```python
from build123d import *

# Parameters (mm, degrees)
SKETCH1_R           = 0.9
BOSS_EXTRUDE1_DEPTH = 2


with BuildPart() as part:
    # Sketch1 → Boss-Extrude1 (new body)
    with BuildSketch(Plane.XY):
        with BuildLine():
            Line((16.2, 5), (16.2, 2))
            ThreePointArc((16.2, 2), (15.614213562, 0.585786438), (14.2, 0))
            Line((14.2, 0), (2, 0))
            ThreePointArc((2, 0), (0.585786438, 0.585786438), (0, 2))
            Line((0, 2), (0, 5))
            Line((0, 5), (4, 5))
            Line((4, 5), (4, 7))
            Line((4, 7), (0, 7))
            Line((0, 7), (0, 16.525))
            Line((0, 16.525), (4, 16.525))
            Line((4, 16.525), (4, 18.525))
            Line((4, 18.525), (0, 18.525))
            Line((0, 18.525), (0, 21.525))
            ThreePointArc((0, 21.525), (0.585786438, 22.939213562), (2, 23.525))
            Line((2, 23.525), (14.2, 23.525))
            ThreePointArc((14.2, 23.525), (15.614213562, 22.939213562), (16.2, 21.525))
            Line((16.2, 21.525), (16.2, 18.525))
            Line((16.2, 18.525), (12.2, 18.525))
            Line((12.2, 18.525), (12.2, 16.525))
            Line((12.2, 16.525), (16.2, 16.525))
            Line((16.2, 16.525), (16.2, 7))
            Line((16.2, 7), (12.2, 7))
            Line((12.2, 7), (12.2, 5))
            Line((12.2, 5), (16.2, 5))
        make_face()
        with Locations((13.45, 2.5)):
            Circle(SKETCH1_R, mode=Mode.SUBTRACT)
        with Locations((2.75, 21.025)):
            Circle(SKETCH1_R, mode=Mode.SUBTRACT)
        with Locations((13.45, 21.025)):
            Circle(SKETCH1_R, mode=Mode.SUBTRACT)
        with Locations((2.75, 2.5)):
            Circle(SKETCH1_R, mode=Mode.SUBTRACT)
    extrude(amount=BOSS_EXTRUDE1_DEPTH)


solid = part.part
```
Could you check a few things on this model? Use its own coordinates, in mm. A direction names the side the tool comes from. Coordinates: 2 decimals unless noted, no trailing zeros. Write each loop counter-clockwise with the first axis right and the second up, starting at its lowest first coordinate (ties: lowest second). Pieces come first, ordered by that corner, then holes. Notation, with made-up numbers: (48, 11) -> (65, 11) arc R27 cw to (65, 34) -> close; hole circle Ø11 at (89, -23.5). An arc over 180 degrees is marked (long way). Write item = value, one per line. Start each with the question number.
(1) I want a section at A-A (x = 2.75). Please give me the cut outline in (y, z) (3 decimals).
(2) Will this pin go through, and if not, where does the flat tip stop? pin 1 (0.6 mm diameter, centred on x = 15, z = 1, fed in from -Y).
(3) I need wall thicknesses on line 1 (Y direction, x = 13.45, z = 1.05) (3 decimals); line 2 (X direction, y = 20.5, z = 0.8); line 3 (Y direction, x = 3.5, z = 1.8) (1 decimal). Which ranges of each line are inside material? Lowest first, please. Write a range as [from, to].
(4) We'd pull the mould along X, two halves only. Please class faces 4 (the face through (2, 5, 1)), 5 (the face through (4, 18, 1)), 6 (the face through (12.2, 6, 1)), 7 (the face through (14.3, 2.2, 1)): released by +X, released by -X, zero draft, split by the parting line, or undercut.
(5) I want a section at D-D (x = 15). Please give me the cut outline in (y, z) (3 decimals), plus the area to 3 significant figures.
(6) Which directions (+Z, -Z, +X, -X, +Y, -Y) give clear straight access to the entire face, cutting with the end or side of a thin tool? Please do faces 1 (the face through (0.57, 22.924, 0.986)), 2 (the face through (2, 18.525, 1)), 3 (the face through (14, 16.525, 1)).
(7) I want a section at B-B (y = 2.5). Please give me the cut outline in (x, z).
(8) I want a section at C-C (z = 1.1). Please give me the cut outline in (x, y) (3 decimals).
Result set:
q1.outline = (0, 0) -> (1.6, 0) -> (1.6, 2) -> (0, 2) -> close; (3.4, 0) -> (5, 0) -> (5, 2) -> (3.4, 2) -> close; (7, 0) -> (16.525, 0) -> (16.525, 2) -> (7, 2) -> close; (18.525, 0) -> (20.125, 0) -> (20.125, 2) -> (18.525, 2) -> close; (21.925, 0) -> (23.525, 0) -> (23.525, 2) -> (21.925, 2) -> close
q2.pin_1 = 0.06
q3.line_1 = [0, 1.6], [3.4, 5], [7, 16.525], [18.525, 20.125], [21.925, 23.525]
q3.line_2 = [0, 2.02], [3.48, 12.72], [14.18, 16.2]
q3.line_3 = [0, 2], [3, 5], [7, 16.5], [18.5, 20.5], [21.5, 23.5]
q4.face_4 = zero draft
q4.face_5 = released by -X
q4.face_6 = released by +X
q4.face_7 = undercut
q5.outline = (0.167, 0) -> (5, 0) -> (5, 2) -> (0.167, 2) -> close; (7, 0) -> (16.525, 0) -> (16.525, 2) -> (7, 2) -> close; (18.525, 0) -> (23.358, 0) -> (23.358, 2) -> (18.525, 2) -> close
q5.area = 38.4 mm2
q6.face_1 = +Z, -Z, -X, +Y
q6.face_2 = +Z, -Z, -X
q6.face_3 = +Z, -Z, +X
q7.outline = (0, 0) -> (1.85, 0) -> (1.85, 2) -> (0, 2) -> close; (3.65, 0) -> (12.55, 0) -> (12.55, 2) -> (3.65, 2) -> close; (14.35, 0) -> (16.2, 0) -> (16.2, 2) -> (14.35, 2) -> close
q8.outline = (0, 2) arc R2 ccw to (2, 0) -> (14.2, 0) arc R2 ccw to (16.2, 2) -> (16.2, 5) -> (12.2, 5) -> (12.2, 7) -> (16.2, 7) -> (16.2, 16.525) -> (12.2, 16.525) -> (12.2, 18.525) -> (16.2, 18.525) -> (16.2, 21.525) arc R2 ccw to (14.2, 23.525) -> (2, 23.525) arc R2 ccw to (0, 21.525) -> (0, 18.525) -> (4, 18.525) -> (4, 16.525) -> (0, 16.525) -> (0, 7) -> (4, 7) -> (4, 5) -> (0, 5) -> close; hole circle Ø1.8 at (2.75, 2.5); hole circle Ø1.8 at (2.75, 21.025); hole circle Ø1.8 at (13.45, 2.5); hole circle Ø1.8 at (13.45, 21.025)
